Source: CAD feature listing. Evaluate the final solid. Frame: model axes, mm. A direction names the side the tool comes from. Coordinates: 2 decimals unless noted, no trailing zeros. Write each loop counter-clockwise with the first axis right and the second up, starting at its lowest first coordinate (ties: lowest second). Pieces come first, ordered by that corner, then holes. Notation, with made-up numbers: M 45,12.5 L 76,12.5 A10 cw 76,20.5 Z; hole C 77,22.25 d10. An arc over 180 degrees is marked long. Answer as CSV lines item,"result". Start each with the question number.
1. Section B-B on y = -11.5. Return the cut outline in (x, z).
2. Section D-D on y = -31.5. Return the cut outline in (x, z), plus the area to 3 significant figures.
3. Mould query, pull axis Z, two halves, no side actions, for faces 5 (the face through (-36.72, -11.05, -0.43)), 6 (the face through (-60, -35, -26)), 7 (the face through (-1, -35, -30)). Classes: pulls with the +Z half, pulls with the -Z half, needs draft (parallel to the pull), parting line crosses it, or undercut.
4. Section A-A on y = -5. Return the cut outline in (x, z).
5. Contact query for flat-ended pins moving along their axis: pin 1 Ø6 at (x, y) = (27.5, -7.5) entering from +Z; pin 2 Ø2 at (y, z) = (-31, 15) entering from -X; pin 3 Ø8 at (x, z) = (3, -4) entering from +Y; pin 4 Ø9 at (x, y) = (13.5, -16) entering from -Z. Output: stop coordinate, or through.
6. Line query: probe 1 along X at (y, z) = (-16.75, 0); probe 2 along Y at (x, z) = (27, 27); probe 3 along X at (y, z) = (-12.5, 1). Output: solid intervals per line, ascending. Write a range as [from, to].
7. Reachability of faces 1 (the face through (-53, -35, 22.5)), 2 (the face through (50, -15, 0)), 3 (the face through (53, -35, 22.5)), 4 (the face through (0, -34, 0)) from +Z, -Z, +X, -X, +Y, -Y: full face, straight path, thin tool, end or side. Return the list, or none.
```python
from build123d import *

# Parameters (mm, degrees)
EXTRUDE_2_DEPTH          = 19
EXTRUDE_5_DEPTH          = 40
CUT_EXTRUDE_START        = -10
SKETCH_1_4_R             = 24
CUT_EXTRUDE_1_DEPTH      = 20
SKETCH_4_W               = 120
SKETCH_4_H               = 60
EXTRUDE_6_DEPTH          = 10
FILLET_2_R               = 5
CUT_EXTRUDE_2_DEPTH      = 79.102496759
MIRROR_2_COPY_1_DEPTH    = 79.102496759
CUT_EXTRUDE_3_DEPTH      = 12
SKETCH_6_W               = 25
SKETCH_6_H               = 6
CUT_EXTRUDE_4_DEPTH      = 12
FILLET_3_R               = 4
FILLET_4_R               = 2
SKETCH_7_R               = 3.3095
CUT_EXTRUDE_5_DEPTH      = 25
CHAMFER_1_SIZE           = 3.3
CHAMFER_2_SIZE           = 0.6905
SKETCH_11_W              = 120
SKETCH_11_H              = 68
CUT_EXTRUDE_8_DEPTH      = 80.724525712
CUT_EXTRUDE_9_DEPTH      = 90.493016487
CUT_EXTRUDE_9_DEPTH_BACK = 9
SKETCH_12_W              = 80
SKETCH_12_H              = 30
SKETCH_13_W              = 80
SKETCH_13_H              = 30
CUT_EXTRUDE_10_DEPTH     = 83.462112512


with BuildPart() as part:
    # Эскиз1 → Бобышка-Вытянуть2 (new, symmetric)
    with BuildSketch(Plane.XY):
        with BuildLine():
            Line((35, 0), (26, 0))
            ThreePointArc((26, 0), (0, -26), (-26, 0))
            Line((-26, 0), (-35, 0))
            ThreePointArc((-35, 0), (0, -35), (35, 0))
        make_face()
        with BuildLine():
            Line((26, 0), (24, 0))
            ThreePointArc((24, 0), (0, -24), (-24, 0))
            Line((-24, 0), (-26, 0))
            ThreePointArc((-26, 0), (0, -26), (26, 0))
        make_face()
    extrude(amount=EXTRUDE_2_DEPTH, both=True)

    # Эскиз2 → Бобышка-Вытянуть5 (add)
    with BuildSketch(Plane(origin=(0, 0, 0), x_dir=(1, 0, 0), z_dir=(0, 1, 0))):
        with BuildLine():
            Line((-40, 10), (40, 10))
            ThreePointArc((40, 10), (50, 0), (40, -10))
            Line((40, -10), (-40, -10))
            ThreePointArc((-40, -10), (-50, 0), (-40, 10))
        make_face()
    extrude(amount=-EXTRUDE_5_DEPTH)

    # Эскиз1<4> → Вырез-Вытянуть1 (cut)
    with BuildSketch(Plane.XY.offset(CUT_EXTRUDE_START)):
        Circle(SKETCH_1_4_R)
    extrude(amount=CUT_EXTRUDE_1_DEPTH, mode=Mode.SUBTRACT)

    # Эскиз4 → Бобышка-Вытянуть6 (add)
    with BuildSketch(Plane.XZ.offset(40)):
        Rectangle(SKETCH_4_W, SKETCH_4_H)
    extrude(amount=-EXTRUDE_6_DEPTH)

    # Скругление2
    fillet_2_edges = [part.edges().sort_by_distance(p)[0] for p in [
        (-18.027756377, -30, 14.5),
        (18.027756377, -30, 14.5),
        (18.027756377, -30, -14.5),
        (-18.027756377, -30, -14.5),
    ]]
    fillet(fillet_2_edges, radius=FILLET_2_R)

    # Эскиз5 → Вырез-Вытянуть2 (cut, through all)
    with BuildSketch(Plane.XZ.offset(40)):
        with BuildLine():
            Line((75, -22.5), (45, -22.5))
            ThreePointArc((45, -22.5), (40, -17.5), (45, -12.5))
            Line((45, -12.5), (75, -12.5))
            ThreePointArc((75, -12.5), (80, -17.5), (75, -22.5))
        make_face()
    cut_extrude_2 = extrude(amount=-CUT_EXTRUDE_2_DEPTH, mode=Mode.SUBTRACT)

    # Зеркальное отражение1: Вырез-Вытянуть2 across plane
    add(cut_extrude_2.mirror(Plane.XY), mode=Mode.SUBTRACT)

    # Зеркальное отражение2: Вырез-Вытянуть2 across plane
    add(cut_extrude_2.mirror(Plane(origin=(0, 0, 0), x_dir=(0, 0, 1), z_dir=(1, 0, 0))), mode=Mode.SUBTRACT)

    # Зеркальное отражение2 copy 1 sketch → Зеркальное отражение2 copy 1 (cut, through all)
    with BuildSketch(Plane(origin=(0, -40, 0), x_dir=(-1, 0, 0), z_dir=(0, -1, 0))):
        with BuildLine():
            Line((75, -22.5), (45, -22.5))
            ThreePointArc((45, -22.5), (40, -17.5), (45, -12.5))
            Line((45, -12.5), (75, -12.5))
            ThreePointArc((75, -12.5), (80, -17.5), (75, -22.5))
        make_face()
    extrude(amount=-MIRROR_2_COPY_1_DEPTH, mode=Mode.SUBTRACT)

    # Эскиз1<5> → Вырез-Вытянуть3 (cut, symmetric)
    with BuildSketch(Plane.XY):
        with BuildLine():
            ThreePointArc((-24, 0), (0, 24), (24, 0))
            Line((24, 0), (26, 0))
            ThreePointArc((26, 0), (0, 26), (-26, 0))
            Line((-26, 0), (-24, 0))
        make_face()
        with BuildLine():
            Line((26, 0), (24, 0))
            ThreePointArc((24, 0), (0, -24), (-24, 0))
            Line((-24, 0), (-26, 0))
            ThreePointArc((-26, 0), (0, -26), (26, 0))
        make_face()
    extrude(amount=CUT_EXTRUDE_3_DEPTH, both=True, mode=Mode.SUBTRACT)

    # Эскиз6 → Вырез-Вытянуть4 (cut, symmetric)
    with BuildSketch(Plane.XY):
        with Locations((12.5, -37)):
            Rectangle(SKETCH_6_W, SKETCH_6_H)
    cut_extrude_4 = extrude(amount=CUT_EXTRUDE_4_DEPTH, both=True, mode=Mode.SUBTRACT)

    # Зеркальное отражение3: Вырез-Вытянуть4 across plane
    add(cut_extrude_4.mirror(Plane(origin=(0, -34, -12), x_dir=(0, 0, 1), z_dir=(-1, 0, 0))), mode=Mode.SUBTRACT)

    # Скругление3
    fillet_3_edges = [part.edges().sort_by_distance(p)[0] for p in [
        (25, -34, 0),
        (-25, -34, 0),
    ]]
    fillet(fillet_3_edges, radius=FILLET_3_R)

    # Скругление4
    fillet_4_edges = [part.edges().sort_by_distance(p)[0] for p in [
        (-23.828427125, -35.171572875, 12),
        (23.828427125, -35.171572875, 12),
        (-23.828427125, -35.171572875, -12),
        (23.828427125, -35.171572875, -12),
        (0, -34, 12),
        (0, -34, -12),
        (0, -40, 12),
        (-25, -40, 0),
        (25, -40, 0),
        (0, -40, -12),
    ]]
    fillet(fillet_4_edges, radius=FILLET_4_R - 0.0001)  # a hair under: the kernel refuses the full size

    # Эскиз7 → Вырез-Вытянуть5 (cut)
    with BuildSketch(Plane(origin=(0, 0, 0), x_dir=(1, 0, 0), z_dir=(0, 1, 0))):
        with Locations(Location((-40, 0, 0), (0, 0, 270))):
            Circle(SKETCH_7_R)
        with Locations(Location((40, 0, 0), (0, 0, 270))):
            Circle(SKETCH_7_R)
    extrude(amount=-CUT_EXTRUDE_5_DEPTH, mode=Mode.SUBTRACT)

    # Фаска1
    chamfer_1_edges = [part.edges().sort_by_distance(p)[0] for p in [
        (-40, -25, -3.3095),
        (40, -25, -3.3095),
    ]]
    chamfer(chamfer_1_edges, length=CHAMFER_1_SIZE)

    # Фаска2
    chamfer_2_edges = [part.edges().sort_by_distance(p)[0] for p in [
        (-40, 0, -3.3095),
        (40, 0, -3.3095),
    ]]
    chamfer(chamfer_2_edges, length=CHAMFER_2_SIZE)

    # Эскиз8 → Повернуть1 (revolve)
    with BuildSketch(Plane.XY):
        with BuildLine():
            Line((0, 34), (0, -34))
            ThreePointArc((0, -34), (-34, 0), (0, 34))
        make_face()
    revolve(axis=Axis((0, 0, 0), (0, 1, 0)))

    # Эскиз9 → Вырез-Повернуть1 (revolve, cut)
    with BuildSketch(Plane.XY):
        with BuildLine():
            Line((0, 29), (0, -29))
            ThreePointArc((0, -29), (-29, 0), (0, 29))
        make_face()
    revolve(axis=Axis((0, 0, 0), (0, 1, 0)), mode=Mode.SUBTRACT)

    # Эскиз11 → Вырез-Вытянуть8 (cut, through all)
    with BuildSketch(Plane(origin=(0, 0, 0), x_dir=(1, 0, 0), z_dir=(0, 1, 0))):
        Rectangle(SKETCH_11_W, SKETCH_11_H)
    extrude(amount=CUT_EXTRUDE_8_DEPTH, mode=Mode.SUBTRACT)

    # Эскиз12 → Вырез-Вытянуть9 (cut, two sides: drawn at the far end of the back side and taken through both)
    with BuildSketch(Plane.XY.offset(19).offset(-CUT_EXTRUDE_9_DEPTH_BACK)):
        with Locations((0, -15)):
            Rectangle(SKETCH_12_W, SKETCH_12_H)
    extrude(amount=CUT_EXTRUDE_9_DEPTH + CUT_EXTRUDE_9_DEPTH_BACK, mode=Mode.SUBTRACT)

    # Эскиз13 → Вырез-Вытянуть10 (cut, through all)
    with BuildSketch(Plane(origin=(0, 0, -10), x_dir=(-1, 0, 0), z_dir=(0, 0, -1))):
        with Locations((0, -15)):
            Rectangle(SKETCH_13_W, SKETCH_13_H)
    extrude(amount=CUT_EXTRUDE_10_DEPTH, mode=Mode.SUBTRACT)


solid = part.part
```
Values:
1,outline,"M -40,-10 L -24.67,-10 A26.62 cw -24.67,10 L -40,10 A10 ccw Z; M 24.67,-10 L 40,-10 A10 ccw 40,10 L 24.67,10 A26.62 cw Z; hole C -40,0 d6.62; hole C 40,0 d6.62"
2,outline,"M -60,-30 L 60,-30 L 60,-22.5 L 45,-22.5 A5 cw 45,-12.5 L 60,-12.5 L 60,12.5 L 45,12.5 A5 cw 45,22.5 L 60,22.5 L 60,30 L -60,30 L -60,22.5 L -45,22.5 A5 cw -45,12.5 L -60,12.5 L -60,-12.5 L -45,-12.5 A5 cw -45,-22.5 L -60,-22.5 Z"
2,area,"6,440 mm²"
3,face 5,"undercut"
3,face 6,"needs draft"
3,face 7,"pulls with the -Z half"
4,outline,"M -40,-10 L -26.76,-10 A28.57 cw -26.76,10 L -40,10 A10 ccw Z; M 26.76,-10 L 40,-10 A10 ccw 40,10 L 26.76,10 A28.57 cw Z; hole C -40,0 d6.62; hole C 40,0 d6.62"
5,pin 1,"z = 10"
5,pin 2,"x = -41.43"
5,pin 3,"y = -27.57"
5,pin 4,"through"
6,probe 1,"[-50, -43.31], [-36.69, -23.67], [23.67, 36.69], [43.31, 50]"
6,probe 2,"[-40, -30]"
6,probe 3,"[-49.95, -43.15], [-36.85, -26.15], [26.15, 36.85], [43.15, 49.95]"
7,face 1,"-X, +Y, -Y"
7,face 2,"+X, +Y"
7,face 3,"+X, +Y, -Y"
7,face 4,"-Y"
